Source: CAD feature listing. Evaluate the final solid. Frame: model axes, mm. A direction names the side the tool comes from. Round coordinates to 2 decimals unless told otherwise and drop trailing zeros. Loops run counter-clockwise (first coordinate to the right, second up) from the corner with the lowest first, then second, coordinate; pieces in that order, holes last. Notation, with made-up numbers: M -35.5,-9.75 L -30.5,-9.75 A15 ccw -30.5,5.25 Z; hole C -25.75,-17 d6. An arc over 180 degrees is marked long. One line per item, written item: value.
from build123d import *

# Parameters (mm, degrees)
SALIENTE_EXTRUIR1_DEPTH = 10


with BuildPart() as part:
    # Croquis1 → Saliente-Extruir1 (new body)
    with BuildSketch(Plane.XY):
        with BuildLine():
            Line((-13.75, 0), (13.75, 0))
            ThreePointArc((13.75, 0), (17.762966925, 1.443448089), (19.937041964, 5.11235033))
            Line((19.937041964, 5.11235033), (27.765257697, 45.893315022))
            ThreePointArc((27.765257697, 45.893315022), (26.949859086, 50.156238741), (23.428875228, 52.693967294))
            Line((23.428875228, 52.693967294), (14.23949707, 55))
            Line((14.23949707, 55), (8.642217346, 25.841060779))
            ThreePointArc((8.642217346, 25.841060779), (0, 18.7), (-8.642217346, 25.841060779))
            Line((-8.642217346, 25.841060779), (-14.23949707, 55))
            Line((-14.23949707, 55), (-23.428875228, 52.693967294))
            ThreePointArc((-23.428875228, 52.693967294), (-26.949859086, 50.156238741), (-27.765257697, 45.893315022))
            Line((-27.765257697, 45.893315022), (-19.937041964, 5.11235033))
            ThreePointArc((-19.937041964, 5.11235033), (-17.762966925, 1.443448089), (-13.75, 0))
        make_face()
    extrude(amount=SALIENTE_EXTRUIR1_DEPTH)


solid = part.part
1. Section query D-D (x = 6.5). Return the cut outline in (y, z), and give its area (3 significant figures).
Report:
outline: M 0,0 L 21.57,0 L 21.57,10 L 0,10 Z
area: 216 mm2
2. Ray query, line 1 (X direction, y = 43, z = 4.75); line 2 (X direction, y = 38, z = 6.5); line 3 (Y direction, x = -5.5, z = 6.75). Return the intervals inside material, ascending. Write a range as [from, to].
Report:
line 1: x = [-27.21, -11.94], [11.94, 27.21]
line 2: x = [-26.25, -10.98], [10.98, 26.25]
line 3: y = [0, 20.63]
3. Section query C-C (y = 20). Return the cut outline in (x, z).
Report:
outline: M -22.79,0 L -4.6,0 L -4.6,10 L -22.79,10 Z; M 4.6,0 L 22.79,0 L 22.79,10 L 4.6,10 Z
4. Reachability of faces 4 (the face through (0, 16, 10)), 5 (the face through (-11.4, 40.2, 4.9)) from +Z, -Z, +X, -X, +Y, -Y: full face, straight path, thin tool, end or side. Return the list, or none.
Report:
face 4: +Z, +X, -X, +Y, -Y
face 5: +Z, -Z, +Y
5. Section query A-A (y = 28). Return the cut outline in (x, z).
Report:
outline: M -24.33,0 L -9.06,0 L -9.06,10 L -24.33,10 Z; M 9.06,0 L 24.33,0 L 24.33,10 L 9.06,10 Z
6. Section query B-B (z = 6). Return the cut outline in (x, y).
Report:
outline: M -27.77,45.89 L -19.94,5.11 A6.3 ccw -13.75,0 L 13.75,0 A6.3 ccw 19.94,5.11 L 27.77,45.89 A5.87 ccw 23.43,52.69 L 14.24,55 L 8.64,25.84 A8.8 cw -8.64,25.84 L -14.24,55 L -23.43,52.69 A5.87 ccw Z
7. Pull-direction query (X, two-part tool) for faces 1 (the face through (-26.916, 50.209, 4.93)), 2 (the face through (23.796, 25.217, 4.93)), 3 (the face through (11.48, 40.62, 4.93)); classes: released by +X, released by -X, zero draft, split by the parting line, or undercut.
Report:
face 1: released by -X
face 2: released by +X
face 3: undercut
8. Pin query (flat end, axial travel): pin 1 (3 mm diameter, centred on x = -19.5, z = 1.5, fed in from +Y); pin 2 (3 mm diameter, centred on y = 42.5, z = 7, fed in from +X); pin 3 (3 mm diameter, centred on x = -17, z = 5, fed in from +Y). Return the tip coordinate at first contact, or that it passes through.
Report:
pin 1: stops at y = 54.06
pin 2: stops at x = 27.4
pin 3: stops at y = 54.68
